from build123d import *

# Parameters (mm, degrees)
BOSS_EXTRUDE1_DEPTH = 2.032
FILLET1_R           = 2
SKETCH4_R           = 1.2446
CUT_EXTRUDE1_DEPTH  = 75.115872934


with BuildPart() as part:
    # Sketch3 → Boss-Extrude1 (new body)
    with BuildSketch(Plane.XY):
        with BuildLine():
            Line((62.980794963, 30.66873734), (50.569205037, 30.66873734))
            ThreePointArc((50.569205037, 30.66873734), (45.275, 28.075), (39.980794963, 30.66873734))
            Line((39.980794963, 30.66873734), (27.569205037, 30.66873734))
            ThreePointArc((27.569205037, 30.66873734), (22.275, 28.075), (16.980794963, 30.66873734))
            Line((16.980794963, 30.66873734), (10.658308864, 17.473983742))
            ThreePointArc((10.658308864, 17.473983742), (13.670205209, 16.817167392), (16.069205037, 14.88126266))
            Line((16.069205037, 14.88126266), (28.480794963, 14.88126266))
            ThreePointArc((28.480794963, 14.88126266), (33.775, 17.475), (39.069205037, 14.88126266))
            Line((39.069205037, 14.88126266), (51.480794963, 14.88126266))
            ThreePointArc((51.480794963, 14.88126266), (56.775, 17.475), (62.069205037, 14.88126266))
            Line((62.069205037, 14.88126266), (68.391691136, 28.076016258))
            ThreePointArc((68.391691136, 28.076016258), (65.379794791, 28.732832608), (62.980794963, 30.66873734))
        make_face()
    extrude(amount=BOSS_EXTRUDE1_DEPTH)

    # Fillet1
    fillet1_edges = [part.edges().sort_by_distance(p)[0] for p in [
        (68.391691136, 28.076016258, 1.016),
        (62.069205037, 14.88126266, 1.016),
        (51.480794963, 14.88126266, 1.016),
        (39.069205037, 14.88126266, 1.016),
        (28.480794963, 14.88126266, 1.016),
        (16.069205037, 14.88126266, 1.016),
        (10.658308864, 17.473983742, 1.016),
        (16.980794963, 30.66873734, 1.016),
        (27.569205037, 30.66873734, 1.016),
        (39.980794963, 30.66873734, 1.016),
        (50.569205037, 30.66873734, 1.016),
        (62.980794963, 30.66873734, 1.016),
    ]]
    fillet(fillet1_edges, radius=FILLET1_R)

    # Sketch4 → Cut-Extrude1 (cut, through all)
    with BuildSketch(Plane.XY.offset(2.032)):
        with Locations((22.275, 20.49206771)):
            Circle(SKETCH4_R)
        with Locations((56.775, 25.05793229)):
            Circle(SKETCH4_R)
    extrude(amount=-CUT_EXTRUDE1_DEPTH, mode=Mode.SUBTRACT)


solid = part.part
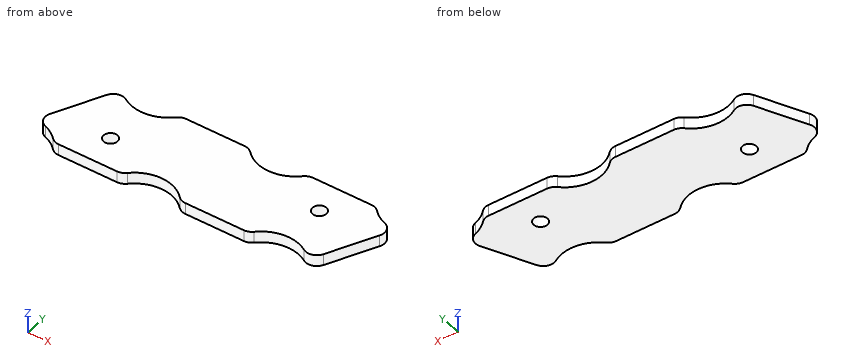
Work out the finished part from the listing and answer in its coordinate system (mm). Give positions to 0.01 mm unless a question says otherwise; leave off trailing zeros. Loops run counter-clockwise (first coordinate to the right, second up) from the corner with the lowest first, then second, coordinate; pieces in that order, holes last. Notation, with made-up numbers: (50.25, 72) - (58.25, 72) arc R9 ccw to (58.25, 83) - close; hole circle Ø8 at (39, 7). An arc over 180 degrees is marked (long way). Answer in a Markdown table with one row per item.
(1) Flat-ended cylindrical pins translate along their axes: pin 1 Ø1 at (y, z) = (25.5, 1.5) entering from -X; pin 2 Ø1 at (y, z) = (25.5, 1) entering from +X; pin 3 Ø1 at (y, z) = (17, 0.5) entering from +X. Find the tip coordinate at first contact, or state that the pin passes through.
Results list:
| item | result |
|---|---|
| pin 1 | stops at x = 14.26 |
| pin 2 | stops at x = 67.37 |
| pin 3 | stops at x = 63.32 |
(2) Section B-B (x = 30) is taken. Give the vertices of the cut face in (y, z).
Results list:
| item | result |
|---|---|
| outline | (16.31, 0) - (30.67, 0) - (30.67, 2.03) - (16.31, 2.03) - close |
(3) Section A-A (z = 0.6) is taken. Give the vertices of the cut face in (x, y) (3 decimals), and give its area (3 significant figures).
Results list:
| item | result |
|---|---|
| outline | (11.804, 19.865) arc R2 ccw to (12.957, 17.11) arc R6.7 cw to (15.547, 15.478) arc R2 ccw to (16.972, 14.881) - (27.578, 14.881) arc R2 ccw to (29.003, 15.478) arc R6.7 cw to (38.547, 15.478) arc R2 ccw to (39.972, 14.881) - (50.578, 14.881) arc R2 ccw to (52.003, 15.478) arc R6.7 cw to (60.346, 16.444) arc R2 ccw to (63.215, 17.272) - (67.246, 25.685) arc R2 ccw to (66.093, 28.44) arc R6.7 cw to (63.503, 30.072) arc R2 ccw to (62.078, 30.669) - (51.472, 30.669) arc R2 ccw to (50.047, 30.072) arc R6.7 cw to (40.503, 30.072) arc R2 ccw to (39.078, 30.669) - (28.472, 30.669) arc R2 ccw to (27.047, 30.072) arc R6.7 cw to (18.704, 29.106) arc R2 ccw to (15.835, 28.278) - close; hole circle Ø2.489 at (22.275, 20.492); hole circle Ø2.489 at (56.775, 25.058) |
| area | 715 mm² |
(4) Section C-C (y = 22.25) is taken. Give the vertices of the cut face in (x, z), and give its area (3 significant figures).
Results list:
| item | result |
|---|---|
| outline | (12.95, 0) - (65.6, 0) - (65.6, 2.03) - (12.95, 2.03) - close |
| area | 107 mm² |
(5) Consider L1, parallel to Y at x = 34, z = 0.6; L2, parallel to X at y = 21.5, z = 1.4; L3, parallel to X at y = 16.5, z = 1.55. Determine where each line is inside the solid, lowest interval first. Write a range as [from, to].
Results list:
| item | result |
|---|---|
| L1 | y = [17.47, 30.67] |
| L2 | x = [12.59, 21.54], [23.01, 65.24] |
| L3 | x = [14.26, 30.29], [37.26, 53.29], [60.26, 62.56] |
